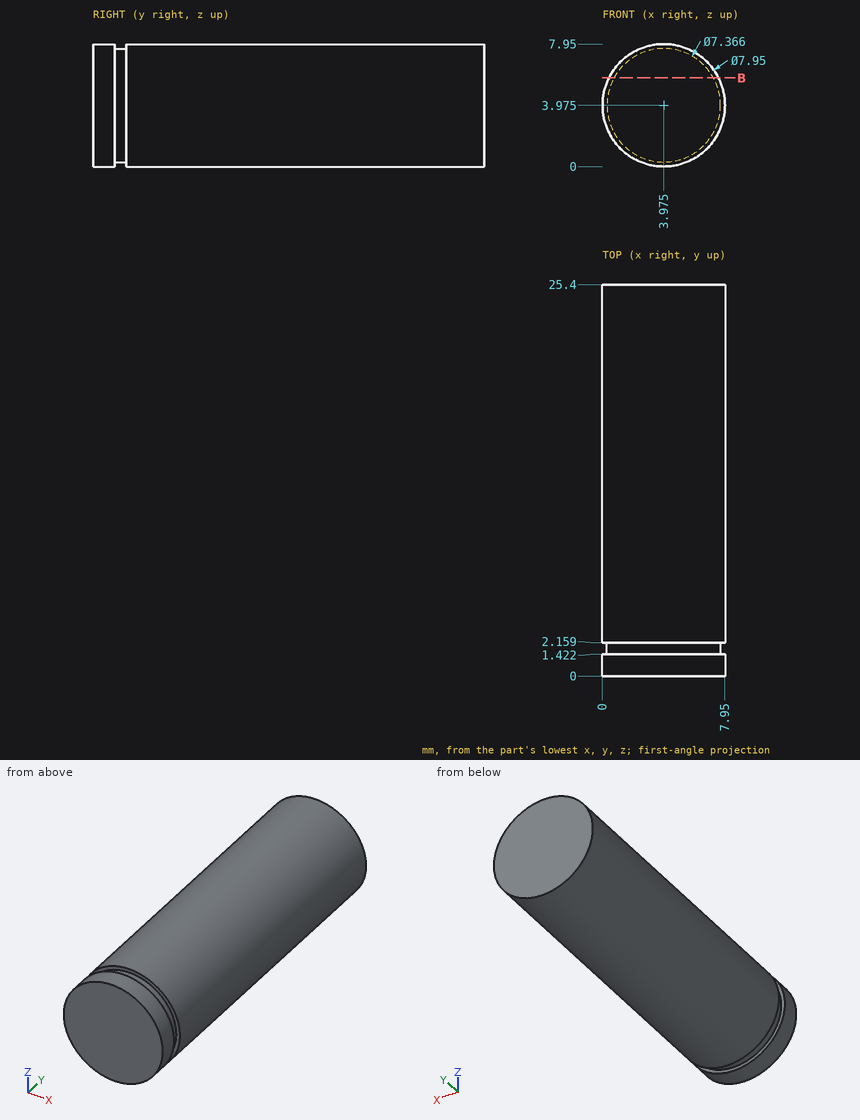
The figure shows three views and two pictorial views of one solid part (mm, origin at its lowest corner). Answer the questions. Give positions to 0.01 mm unless a question says otherwise; leave off trailing zeros. Write each loop counter-clockwise with the first axis right and the second up, starting at its lowest first coordinate (ties: lowest second). Pieces come first, ordered by that corner, then holes.
Q1. Given pin 1 (2 mm diameter, centred on y = 2.5, z = 5.5, fed in from -X) (1 decimal), flat-ended and moving along its own axis, determine where the tip first touches the part or whether it passes through.
Answer:
pin 1: stops at x = 0
Q2. The part is cut by section B-B on z = 5.75. Give the vertices of the cut face in (x, y).
Answer:
outline: (0.42, 0) - (7.53, 0) - (7.53, 1.42) - (7.2, 1.42) - (7.2, 2.16) - (7.53, 2.16) - (7.53, 25.4) - (0.42, 25.4) - (0.42, 2.16) - (0.75, 2.16) - (0.75, 1.42) - (0.42, 1.42) - close
Q3. Straight lines are drawn through the part: L1, parallel to Y at x = 2.75, z = 7.5; L2, parallel to Z at x = 1, y = 3.5; L3, parallel to Z at x = 7.5, y = 21.5 (1 decimal). For each, find the intervals that lie inside material, in ascending order.
Answer:
L1: y = 0 to 1.42, 2.16 to 25.4
L2: z = 1.34 to 6.61
L3: z = 2.1 to 5.8
